Read the model definition and answer for the solid it produces. Units are mm, in the model's axes. Face numbers are marked on the shaded views. Give positions to 0.01 mm unless a question says otherwise; leave off trailing zeros. Write each loop counter-clockwise with the first axis right and the second up, starting at its lowest first coordinate (ties: lowest second). Pieces come first, ordered by that corner, then holes. Notation, with made-up numbers: (28.5, 55.5) -> (48.5, 55.5) arc R21 cw to (48.5, 82.5) -> close; hole circle Ø2 at (84, 36). An arc over 180 degrees is marked (long way). Answer as CSV lines item,"result". Start each with the question number.
1. The part is cut by section C-C, the plane z = -10. Determine the outline of the cut face in (x, y).
2. The part is cut by section B-B, the plane x = 9.5. Determine the outline of the cut face in (y, z), and give its area (3 significant figures).
3. Given pin 1 (1.5 mm diameter, centred on x = -2.5, y = 4, fed in from +Z); pin 2 (4 mm diameter, centred on y = 4.5, z = 6.5, fed in from -X); pin 3 (1.8 mm diameter, centred on x = 9, z = 0, fed in from -Y), each flat-ended and moving along its own axis, determine where each tip first touches the part or whether it passes through.
4. For a pull along Y with two mould halves and no side action, classify the marked faces 1, 2 and 3 as pulls with the +Y half, pulls with the -Y half, needs draft (parallel to the pull), parting line crosses it, or undercut.
5. Find the intervals of material crossed by line 1 (X direction, y = 1, z = 0); line 2 (Y direction, x = 12, z = 1); line 3 (X direction, y = 1, z = -12), in increasing order.
6. The part is cut by section A-A, the plane y = 2.5. Determine the outline of the cut face in (x, z).
7. The part is cut by section D-D, the plane x = -12.5. Determine the outline of the cut face in (y, z), and give its area (3 significant figures).
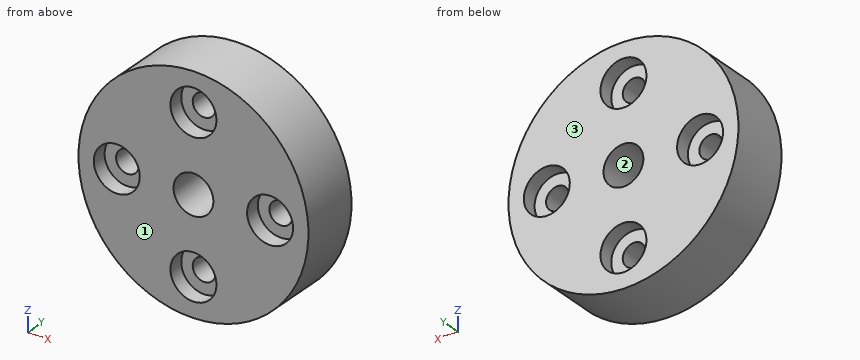
from build123d import *

# Parameters (mm, degrees)
SKETCH1_R           = 15
SKETCH1_R_2         = 1.5
BOSS_EXTRUDE1_DEPTH = 8
SKETCH2_R           = 2.6
CUT_EXTRUDE1_DEPTH  = 23.671568098
CUT_EXTRUDE2_START  = -2
SKETCH3_R           = 3
SKETCH3_R_2         = 1.5
CUT_EXTRUDE2_DEPTH  = 2
SKETCH4_R           = 3
CUT_EXTRUDE3_DEPTH  = 2


with BuildPart() as part:
    # Sketch1 → Boss-Extrude1 (new body)
    with BuildSketch(Plane(origin=(0, 0, 0), x_dir=(1, 0, 0), z_dir=(0, 1, 0))):
        with Locations(Location((0, 0, 0), (0, 0, 270))):
            Circle(SKETCH1_R)
        with Locations(Location((0, 10, 0), (0, 0, 270))):
            Circle(SKETCH1_R_2, mode=Mode.SUBTRACT)
        with Locations(Location((10, 0, 0), (0, 0, 270))):
            Circle(SKETCH1_R_2, mode=Mode.SUBTRACT)
        with Locations(Location((0, -10, 0), (0, 0, 270))):
            Circle(SKETCH1_R_2, mode=Mode.SUBTRACT)
        with Locations(Location((-10, 0, 0), (0, 0, 270))):
            Circle(SKETCH1_R_2, mode=Mode.SUBTRACT)
    extrude(amount=BOSS_EXTRUDE1_DEPTH)

    # Sketch2 → Cut-Extrude1 (cut, through all)
    with BuildSketch(Plane(origin=(0, 8, 0), x_dir=(1, 0, 0), z_dir=(0, 1, 0))):
        with Locations(Location((0, 0, 0), (0, 0, 270))):
            Circle(SKETCH2_R)
    extrude(amount=-CUT_EXTRUDE1_DEPTH, mode=Mode.SUBTRACT)

    # Sketch3 → Cut-Extrude2 (cut)
    # profile 1 of 4: a face of its own
    with BuildSketch(Plane(origin=(0, 8, 0), x_dir=(1, 0, 0), z_dir=(0, 1, 0)).offset(CUT_EXTRUDE2_START)):
        with Locations(Location((-10, 0, 0), (0, 0, 270))):
            Circle(SKETCH3_R)
        with Locations(Location((-10, 0, 0), (0, 0, 270))):
            Circle(SKETCH3_R_2, mode=Mode.SUBTRACT)
    # profile 2 of 4: a face of its own
    with BuildSketch(Plane(origin=(0, 8, 0), x_dir=(1, 0, 0), z_dir=(0, 1, 0)).offset(CUT_EXTRUDE2_START)):
        with Locations(Location((0, -10, 0), (0, 0, 270))):
            Circle(SKETCH3_R)
        with Locations(Location((0, -10, 0), (0, 0, 270))):
            Circle(SKETCH3_R_2, mode=Mode.SUBTRACT)
    # profile 3 of 4: a face of its own
    with BuildSketch(Plane(origin=(0, 8, 0), x_dir=(1, 0, 0), z_dir=(0, 1, 0)).offset(CUT_EXTRUDE2_START)):
        with Locations(Location((10, 0, 0), (0, 0, 270))):
            Circle(SKETCH3_R)
        with Locations(Location((10, 0, 0), (0, 0, 270))):
            Circle(SKETCH3_R_2, mode=Mode.SUBTRACT)
    # profile 4 of 4: a face of its own
    with BuildSketch(Plane(origin=(0, 8, 0), x_dir=(1, 0, 0), z_dir=(0, 1, 0)).offset(CUT_EXTRUDE2_START)):
        with Locations(Location((0, 10, 0), (0, 0, 270))):
            Circle(SKETCH3_R)
    extrude(amount=CUT_EXTRUDE2_DEPTH, mode=Mode.SUBTRACT)

    # Sketch4 → Cut-Extrude3 (cut)
    with BuildSketch(Plane.XZ):
        with Locations(Location((0, 10, 0), (0, 0, 90))):
            Circle(SKETCH4_R)
        with Locations(Location((10, 0, 0), (0, 0, 90))):
            Circle(SKETCH4_R)
        with Locations(Location((0, -10, 0), (0, 0, 90))):
            Circle(SKETCH4_R)
        with Locations(Location((-10, 0, 0), (0, 0, 90))):
            Circle(SKETCH4_R)
    extrude(amount=-CUT_EXTRUDE3_DEPTH, mode=Mode.SUBTRACT)


solid = part.part
Results found:
1,outline,"(-11.18, 0) -> (-3, 0) -> (-3, 2) -> (-1.5, 2) -> (-1.5, 6) -> (-3, 6) -> (-3, 8) -> (-11.18, 8) -> close; (1.5, 2) -> (3, 2) -> (3, 0) -> (11.18, 0) -> (11.18, 8) -> (3, 8) -> (3, 6) -> (1.5, 6) -> close"
2,outline,"(0, -11.61) -> (8, -11.61) -> (8, -2.96) -> (6, -2.96) -> (6, -1.41) -> (2, -1.41) -> (2, -2.96) -> (0, -2.96) -> close; (0, 2.96) -> (2, 2.96) -> (2, 1.41) -> (6, 1.41) -> (6, 2.96) -> (8, 2.96) -> (8, 11.61) -> (0, 11.61) -> close"
2,area,"151 mm²"
3,pin 1,"stops at z = 14.9"
3,pin 2,"stops at x = -14.31"
3,pin 3,"stops at y = 2"
4,face 1,"pulls with the -Y half"
4,face 2,"needs draft"
4,face 3,"pulls with the +Y half"
5,line 1,"x = -15 to -13, -7 to -2.6, 2.6 to 7, 13 to 15"
5,line 2,"y = 2 to 6"
5,line 3,"x = -9 to -2.24, 2.24 to 9"
6,outline,"circle Ø30 at (0, 0); hole circle Ø3 at (-10, 0); hole circle Ø5.2 at (0, 0); hole circle Ø3 at (0, -10); hole circle Ø3 at (0, 10); hole circle Ø3 at (10, 0)"
7,outline,"(0, -8.29) -> (8, -8.29) -> (8, -1.66) -> (6, -1.66) -> (6, 1.66) -> (8, 1.66) -> (8, 8.29) -> (0, 8.29) -> (0, 1.66) -> (2, 1.66) -> (2, -1.66) -> (0, -1.66) -> close"
7,area,"119 mm²"
